For this review, take the finished solid that the model builds, in its own axes (mm). Coordinates: 2 decimals unless noted, no trailing zeros. Loops run counter-clockwise (first coordinate to the right, second up) from the corner with the lowest first, then second, coordinate; pieces in that order, holes last. Notation, with made-up numbers: M 47.5,88 L 80.5,88 A35 ccw 80.5,123 Z; hole C 20.25,-34 d3. An arc over 180 degrees is marked long. Use one line per item in the form item = value.
```python
from build123d import *

# Parameters (mm, degrees)
F0_W     = 22.5
F0_H     = 10
F1_DEPTH = 10
F3_DEPTH = 25
F4_SIZE  = 5


with BuildPart() as f1:
    # F0 (on Top) → F1 (new body)
    with BuildSketch(Plane.XY):
        Rectangle(F0_W, F0_H)
    extrude(amount=F1_DEPTH)

    # F2 (on face) → F3 (cut)
    with BuildSketch(Plane.XZ.offset(5)):
        with BuildLine():
            ThreePointArc((-7.25, 5), (-8.957107, 5.707107), (-8.25, 4))
            ThreePointArc((-8.25, 4), (-7.542893, 4.292893), (-7.25, 5))
        make_face()
        with BuildLine():
            ThreePointArc((9.25, 5), (7.542893, 5.707107), (8.25, 4))
            ThreePointArc((8.25, 4), (8.957107, 4.292893), (9.25, 5))
        make_face()
    extrude(amount=-F3_DEPTH, mode=Mode.SUBTRACT)

    # F4
    f4_edges = [f1.edges().sort_by_distance(p)[0] for p in [
        (-11.25, 0, 10),
        (11.25, 0, 10),
    ]]
    chamfer(f4_edges, length=F4_SIZE)


solid = f1.part
```
1. For pin 1 Ø3 at (y, z) = (-2.5, 8.5) entering from +X, flat-tipped, find the tip position at first contact; note if it passes through.
Computed values:
pin_1 = 9.25
2. Consider section D-D on x = 8.75. Write out the cut boundary in (y, z), plus the area to 3 significant figures.
Computed values:
outline = M -5,0 L 5,0 L 5,4.13 L -5,4.13 Z; M -5,5.87 L 5,5.87 L 5,7.5 L -5,7.5 Z
area = 57.7 mm2
3. Consider section B-B on y = -1.25. Write out the cut boundary in (x, z).
Computed values:
outline = M -11.25,0 L 11.25,0 L 11.25,5 L 6.25,10 L -6.25,10 L -11.25,5 Z; hole C -8.25,5 d2; hole C 8.25,5 d2
4. Consider section A-A on x = -9. Write out the cut boundary in (y, z), plus the area to 3 significant figures.
Computed values:
outline = M -5,0 L 5,0 L 5,4.34 L -5,4.34 Z; M -5,5.66 L 5,5.66 L 5,7.25 L -5,7.25 Z
area = 59.3 mm2
5. Wall thickness on line 1 along X through (y, z) = (4, 5.75); line 2 along X through (y, z) = (-2.5, 8); line 3 along X through (y, z) = (1.75, 9): over which ranges is each line inside the solid? List them lowest first. Write a range as from..to.
Computed values:
line_1 = -10.5..-8.91, -7.59..7.59, 8.91..10.5
line_2 = -8.25..8.25
line_3 = -7.25..7.25
6. Consider section C-C on z = 8.25. Write out the cut boundary in (x, y), plus the area to 3 significant figures.
Computed values:
outline = M -8,-5 L 8,-5 L 8,5 L -8,5 Z
area = 160 mm2
